Geometry check sheet. Reference: the model listing, model coordinates, mm. A direction names the side the tool comes from. Round coordinates to 2 decimals unless told otherwise and drop trailing zeros. Write each loop counter-clockwise with the first axis right and the second up, starting at its lowest first coordinate (ties: lowest second). Pieces come first, ordered by that corner, then holes. Notation, with made-up numbers: (35, 81) -> (53, 81) arc R7 ccw to (53, 89) -> close; hole circle Ø7 at (-4, 54). An arc over 180 degrees is marked (long way). Use a Markdown table: item, result.
```python
from build123d import *

# Parameters (mm, degrees)
F0_R     = 12.7
F1_DEPTH = 25.4


with BuildPart() as f1:
    # F0 (on Top) → F1 (new body)
    with BuildSketch(Plane.XY):
        Polygon((101.6, -31.75), (101.6, 31.75), (63.5, 31.75), (0, 31.75), (-63.5, 31.75), (-101.6, 31.75), (-101.6, -31.75), align=None)
        with Locations((-76.391645, 0)):
            Circle(F0_R, mode=Mode.SUBTRACT)
        with Locations((-38.291645, 0)):
            Circle(F0_R, mode=Mode.SUBTRACT)
        with Locations((-0.191645, 0)):
            Circle(F0_R, mode=Mode.SUBTRACT)
        with Locations((37.908355, 0)):
            Circle(F0_R, mode=Mode.SUBTRACT)
        with Locations((76.008355, 0)):
            Circle(F0_R, mode=Mode.SUBTRACT)
        Polygon((0, 31.75), (63.5, 31.75), (63.5, 95.25), (-63.5, 95.25), (-63.5, 31.75), align=None)
    extrude(amount=F1_DEPTH)


solid = f1.part
```
(1) Access from +Z, -Z, +X, -X, +Y, -Y to the whole of each face (thin tool, end or side, straight path). Record for faces 4 (the face through (-101.6, 0, 13)), 5 (the face through (-82, 31.75, 13)), 6 (the face through (63.5, 63, 13)).
A:
| item | result |
|---|---|
| face 4 | +Z, -Z, -X, +Y, -Y |
| face 5 | +Z, -Z, -X, +Y |
| face 6 | +Z, -Z, +X, +Y |
(2) Section check D-D on y = 43.5. Record the cut outline in (x, z), plus the area to 3 significant figures.
A:
| item | result |
|---|---|
| outline | (-63.5, 0) -> (63.5, 0) -> (63.5, 25.4) -> (-63.5, 25.4) -> close |
| area | 3,230 mm2 |
(3) Section check C-C on z = 11.5. Record the cut outline in (x, y).
A:
| item | result |
|---|---|
| outline | (-101.6, -31.75) -> (101.6, -31.75) -> (101.6, 31.75) -> (63.5, 31.75) -> (63.5, 95.25) -> (-63.5, 95.25) -> (-63.5, 31.75) -> (-101.6, 31.75) -> close; hole circle Ø25.4 at (-76.39, 0); hole circle Ø25.4 at (-38.29, 0); hole circle Ø25.4 at (-0.19, 0); hole circle Ø25.4 at (37.91, 0); hole circle Ø25.4 at (76.01, 0) |
(4) Release check for a two-part mould opening along Y. For faces 1 (the face through (83, 31.75, 13)), 2 (the face through (63.32, 0.56, 12.52)), 3 (the face through (-1, 33, 0)) record: +Y half, -Y half, draft (parallel to the pull), parting line (faces both ways), or undercut.
A:
| item | result |
|---|---|
| face 1 | +Y half |
| face 2 | undercut |
| face 3 | draft |
(5) Section check B-B on x = 7. Record the cut outline in (y, z), plus the area to 3 significant figures.
A:
| item | result |
|---|---|
| outline | (-31.75, 0) -> (-10.47, 0) -> (-10.47, 25.4) -> (-31.75, 25.4) -> close; (10.47, 0) -> (95.25, 0) -> (95.25, 25.4) -> (10.47, 25.4) -> close |
| area | 2,690 mm2 |
(6) Gauge pin test, flat ends, axial feed: pin 1 Ø3 at (y, z) = (47.5, 12) entering from -X; pin 2 Ø1 at (x, y) = (-65.5, 57) entering from +Z; pin 3 Ø1 at (y, z) = (57.5, 10.5) entering from +X. Record the tip position at first contact, or that the pin passes through.
A:
| item | result |
|---|---|
| pin 1 | stops at x = -63.5 |
| pin 2 | passes through |
| pin 3 | stops at x = 63.5 |
(7) Thickness scan on line 1 (X direction, y = -5.5, z = 19.5); line 2 (X direction, y = 9.5, z = 9.5); line 3 (Y direction, x = -0.5, z = 17). Record the ranges inside material, lowest first.
A:
| item | result |
|---|---|
| line 1 | x = -101.6 to -87.84, -64.94 to -49.74, -26.84 to -11.64, 11.26 to 26.46, 49.36 to 64.56, 87.46 to 101.6 |
| line 2 | x = -101.6 to -84.82, -67.96 to -46.72, -29.86 to -8.62, 8.24 to 29.48, 46.34 to 67.58, 84.44 to 101.6 |
| line 3 | y = -31.75 to -12.7, 12.7 to 95.25 |
(8) Section check A-A on y = 0. Record the cut outline in (x, z).
A:
| item | result |
|---|---|
| outline | (-101.6, 0) -> (-89.09, 0) -> (-89.09, 25.4) -> (-101.6, 25.4) -> close; (-63.69, 0) -> (-50.99, 0) -> (-50.99, 25.4) -> (-63.69, 25.4) -> close; (-25.59, 0) -> (-12.89, 0) -> (-12.89, 25.4) -> (-25.59, 25.4) -> close; (12.51, 0) -> (25.21, 0) -> (25.21, 25.4) -> (12.51, 25.4) -> close; (50.61, 0) -> (63.31, 0) -> (63.31, 25.4) -> (50.61, 25.4) -> close; (88.71, 0) -> (101.6, 0) -> (101.6, 25.4) -> (88.71, 25.4) -> close |
